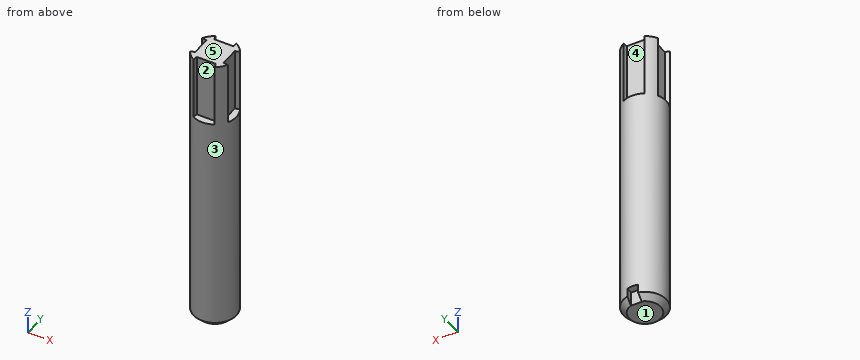
from build123d import *

# Parameters (mm, degrees)
SKETCH1_R           = 9.525
BOSS_EXTRUDE1_DEPTH = 127
SKETCH2_W           = 4.7625
SKETCH2_H           = 3.175
CUT_EXTRUDE1_DEPTH  = 6.35
CHAMFER1_SIZE       = 2.54
CUT_EXTRUDE2_DEPTH  = 27.94


with BuildPart() as part:
    # Sketch1 → Boss-Extrude1 (new body)
    with BuildSketch(Plane.XY):
        Circle(SKETCH1_R)
    extrude(amount=-BOSS_EXTRUDE1_DEPTH)

    # Sketch2 → Cut-Extrude1 (cut)
    with BuildSketch(Plane(origin=(0, 0, -127), x_dir=(-1, 0, 0), z_dir=(0, 0, -1))):
        with Locations((0, 7.9375)):
            Rectangle(SKETCH2_W, SKETCH2_H)
    extrude(amount=-CUT_EXTRUDE1_DEPTH, mode=Mode.SUBTRACT)

    # Chamfer1
    chamfer1_edges = [part.edges().sort_by_distance(p)[0] for p in [
        (-5.83284745, -7.530173678, -127),
    ]]
    chamfer(chamfer1_edges, length=CHAMFER1_SIZE)

    # Sketch3 → Cut-Extrude2 (cut)
    with BuildSketch(Plane.XY):
        with BuildLine():
            Line((-4.720377059, 8.273068682), (-4.064, 6.35))
            Line((-4.064, 6.35), (4.318, 6.35))
            Line((4.318, 6.35), (4.548298042, 8.368907331))
            ThreePointArc((4.548298042, 8.368907331), (-0.098483799, 9.524490849), (-4.720377059, 8.273068682))
        make_face()
        with BuildLine():
            Line((8.273068682, 4.720377059), (6.35, 4.064))
            Line((6.35, 4.064), (6.35, -4.318))
            Line((6.35, -4.318), (8.368907331, -4.548298042))
            ThreePointArc((8.368907331, -4.548298042), (9.524490849, 0.098483799), (8.273068682, 4.720377059))
        make_face()
        with BuildLine():
            Line((4.720377059, -8.273068682), (4.064, -6.35))
            Line((4.064, -6.35), (-4.318, -6.35))
            Line((-4.318, -6.35), (-4.548298042, -8.368907331))
            ThreePointArc((-4.548298042, -8.368907331), (0.098483799, -9.524490849), (4.720377059, -8.273068682))
        make_face()
        with BuildLine():
            Line((-8.273068682, -4.720377059), (-6.35, -4.064))
            Line((-6.35, -4.064), (-6.35, 4.318))
            Line((-6.35, 4.318), (-8.368907331, 4.548298042))
            ThreePointArc((-8.368907331, 4.548298042), (-9.524490849, -0.098483799), (-8.273068682, -4.720377059))
        make_face()
    extrude(amount=-CUT_EXTRUDE2_DEPTH, mode=Mode.SUBTRACT)


solid = part.part
Input: part model. Units: mm. Frame: model coordinates. Face numbers are marked on the shaded views. A direction names the side the tool comes from. Coordinates: 2 decimals unless noted, no trailing zeros. Loops run counter-clockwise (first coordinate to the right, second up) from the corner with the lowest first, then second, coordinate; pieces in that order, holes last. Notation, with made-up numbers: (-6, 64) - (28, 64) arc R33 cw to (28, 96) - close; hole circle Ø8 at (59, 1.25). An arc over 180 degrees is marked (long way). Answer in a Markdown table with one row per item. Add a question column.
Item 1: Section query A-A on y = 0. Return the cut outline in (x, z) (3 decimals).
Item 2: Access query for the marked faces 1 and 2. Directions: +Z, -Z, +X, -X, +Y, -Y. A direction counts if a zero-diameter tool reaches every point of the face in a straight line with its end or side. Return the directions, or none.
Item 3: Line query: line 1 along X through (y, z) = (-8.5, -42.5); line 2 along X through (y, z) = (-0.25, -58); line 3 along Y through (x, z) = (4.75, -72.5). Output: solid intervals per line, ascending. Write a range as [from, to].
Item 4: Section query C-C on z = -110.5. Return the cut outline in (x, y) (3 decimals).
Item 5: Contact query for flat-ended pins moving along their axis: P1, Ø1, axis at y = 7, z = -53.5, coming from the -X side; P2, Ø9, axis at x = 1, z = -8.5, coming from the -Y side; P3, Ø2.5, axis at y = 8.5, z = -123, coming from the +X side. Output: stop coordinate, or through.
Item 6: Section query B-B on x = 0. Return the cut outline in (y, z) (3 decimals), then the cut area to 3 significant figures.
Item 7: Mould query, pull axis X, two halves, no side actions, for the marked faces 3, 4 and 5. Classes: released by +X, released by -X, zero draft, split by the parting line, or undercut.
Recorded:
| question | item | result |
|---|---|---|
| 1 | outline | (-9.525, -124.46) - (-6.985, -127) - (6.985, -127) - (9.525, -124.46) - (9.525, -27.94) - (6.35, -27.94) - (6.35, 0) - (-6.35, 0) - (-6.35, -27.94) - (-9.525, -27.94) - close |
| 2 | face 1 | -Z, +X, -X, +Y, -Y |
| 2 | face 2 | +Z, -Y |
| 3 | line 1 | [-4.3, 4.3] |
| 3 | line 2 | [-9.52, 9.52] |
| 3 | line 3 | [-8.26, 8.26] |
| 4 | outline | circle Ø19.05 at (0, 0) |
| 5 | P1 | x = -6.96 |
| 5 | P2 | y = -8.27 |
| 5 | P3 | x = 6.18 |
| 6 | outline | (-9.525, -124.46) - (-6.985, -127) - (6.35, -127) - (6.35, -120.65) - (9.525, -120.65) - (9.525, -27.94) - (6.35, -27.94) - (6.35, 0) - (-6.35, 0) - (-6.35, -27.94) - (-9.525, -27.94) - close |
| 6 | area | 2,220 mm^2 |
| 7 | face 3 | split by the parting line |
| 7 | face 4 | undercut |
| 7 | face 5 | zero draft |
